from build123d import *

# Parameters (mm, degrees)
REVOLVE2_ANGLE           = 180
SKETCH5_W                = 2.54
SKETCH5_H                = 12.7
SKETCH5_W_2              = 101.6
SKETCH5_H_2              = 2.54
SKETCH5_W_3              = 12.7
BOSS_EXTRUDE1_DEPTH      = 2.54
SKETCH7_W                = 20
SKETCH7_H                = 50
CUT_EXTRUDE1_DEPTH       = 7
BOSS_EXTRUDE3_REACH      = 220.035
SKETCH8_W                = 5
SKETCH8_H                = 91.44
SKETCH9_W                = 6.129296028
SKETCH9_H                = 8.078685473
BOSS_EXTRUDE4_DEPTH      = 2
BOSS_EXTRUDE7_START      = 8
BOSS_EXTRUDE7_DEPTH      = 8
BOSS_EXTRUDE8_REACH      = 220.035
BOSS_EXTRUDE8_END_RADIUS = 40.64
SKETCH13_W               = 75.08
SKETCH13_H               = 60.08
SKETCH13_W_2             = 70
SKETCH13_H_2             = 55
SKETCH14_W               = 75.08
SKETCH14_H               = 60.08
CUT_EXTRUDE3_DEPTH       = 11
BOSS_EXTRUDE9_REACH      = 217.997
SKETCH15_W               = 70
SKETCH15_H               = 55
CUT_EXTRUDE5_DEPTH       = 15
CUT_EXTRUDE6_REACH       = 202.84
SKETCH18_W               = 12
SKETCH18_H               = 56
BOSS_EXTRUDE10_REACH     = 220.035
SKETCH23_W               = 6
SKETCH23_H               = 81.28
SKETCH26_W               = 6
SKETCH26_H               = 53.107211962
BOSS_EXTRUDE11_DEPTH     = 10


with BuildPart() as part:
    # Sketch2 → Revolve2 (revolve)
    with BuildSketch(Plane.XY):
        Polygon((0, 0), (0, 40.64), (0, 45.72), (25.4, 45.72), (195.4, 45.72), (208.1, 45.72), (208.22771659, 40.64), (195.52771659, 40.64), (25.4, 40.64), (5.08, 40.64), (5.08, 0), align=None)
    revolve(axis=Axis((0, 0, 0), (1, 0, 0)), revolution_arc=REVOLVE2_ANGLE)

    # Sketch5 → Boss-Extrude1 (add)
    with BuildSketch(Plane(origin=(0, 0, 0), x_dir=(-1, 0, 0), z_dir=(0, 0, -1))):
        with Locations((-2.54, 34.29)):
            Rectangle(SKETCH5_W, SKETCH5_H)
        with Locations((-104.113858295, -43.18)):
            Rectangle(SKETCH5_W_2, SKETCH5_H_2)
        with Locations((-11.43, 43.18)):
            Rectangle(SKETCH5_W_3, SKETCH5_H_2)
        with Locations((-104.113858295, 43.18)):
            Rectangle(SKETCH5_W_2, SKETCH5_H_2)
        with Locations((-11.43, -43.18)):
            Rectangle(SKETCH5_W_3, SKETCH5_H_2)
        with Locations((-2.54, -34.29)):
            Rectangle(SKETCH5_W, SKETCH5_H)
    extrude(amount=BOSS_EXTRUDE1_DEPTH)

    # Sketch7 → Cut-Extrude1 (cut)
    with BuildSketch(Plane.ZY):
        with Locations((10, 0)):
            Rectangle(SKETCH7_W, SKETCH7_H)
    extrude(amount=-CUT_EXTRUDE1_DEPTH, mode=Mode.SUBTRACT)

    # Sketch8 → Boss-Extrude3 (add, up to next)
    with BuildSketch(Plane(origin=(0, 0, 0), x_dir=(-1, 0, 0), z_dir=(0, 0, -1)), mode=Mode.PRIVATE) as boss_extrude3_sk1:
        with Locations((-15.58, 0)):
            Rectangle(SKETCH8_W, SKETCH8_H)
    boss_extrude3_tool1 = extrude(boss_extrude3_sk1.sketch, amount=-BOSS_EXTRUDE3_REACH, mode=Mode.PRIVATE) - part.part
    add(boss_extrude3_tool1.solids().sort_by_distance((15.58, 0, 0))[0])

    # Sketch9 → Boss-Extrude4 (add)
    with BuildSketch(Plane(origin=(5.08, 0, 0), x_dir=(0, 0, -1), z_dir=(1, 0, 0))):
        with Locations((-3.906446672, 33.952493663)):
            Rectangle(SKETCH9_W, SKETCH9_H)
    extrude(amount=BOSS_EXTRUDE4_DEPTH)

    # Sketch12 → Boss-Extrude7 (add)
    with BuildSketch(Plane.ZY.offset(-13.08).offset(BOSS_EXTRUDE7_START)):
        with BuildLine():
            Line((23.64, 33.056920607), (23.64, -33.056920607))
            ThreePointArc((23.64, -33.056920607), (40.64, 0), (23.64, 33.056920607))
        make_face()
    extrude(amount=-BOSS_EXTRUDE7_DEPTH)

    # Boss-Extrude8: up to this cylinder (the profile starts inside it)
    boss_extrude8_end = Plane(origin=(148.153858, 0, 0), z_dir=(-1, 0, 0)) * Cylinder(BOSS_EXTRUDE8_END_RADIUS, 522.35, mode=Mode.PRIVATE)
    # Sketch13 → Boss-Extrude8 (add, up to the surface)
    with BuildSketch(Plane(origin=(0, 0, 0), x_dir=(-1, 0, 0), z_dir=(0, 0, -1)), mode=Mode.PRIVATE) as boss_extrude8_sk1:
        with Locations((-148.153858295, 0)):
            Rectangle(SKETCH13_W, SKETCH13_H)
        with Locations((-148.153858295, 0)):
            Rectangle(SKETCH13_W_2, SKETCH13_H_2, mode=Mode.SUBTRACT)
    boss_extrude8_tool1 = extrude(boss_extrude8_sk1.sketch, amount=-BOSS_EXTRUDE8_REACH, mode=Mode.PRIVATE) & boss_extrude8_end
    add(boss_extrude8_tool1.solids().sort_by_distance((148.153858, 29.078407, 0))[0])

    # Sketch14 → Cut-Extrude3 (cut)
    with BuildSketch(Plane(origin=(0, 0, 0), x_dir=(-1, 0, 0), z_dir=(0, 0, -1))):
        with Locations((-148.153858295, 0)):
            Rectangle(SKETCH14_W, SKETCH14_H)
    extrude(amount=-CUT_EXTRUDE3_DEPTH, mode=Mode.SUBTRACT)

    # Sketch15 → Boss-Extrude9 (add, up to next)
    with BuildSketch(Plane(origin=(0, 0, 11), x_dir=(-1, 0, 0), z_dir=(0, 0, -1)), mode=Mode.PRIVATE) as boss_extrude9_sk1:
        with Locations((-148.153858295, 0)):
            Rectangle(SKETCH15_W, SKETCH15_H)
    boss_extrude9_tool1 = extrude(boss_extrude9_sk1.sketch, amount=-BOSS_EXTRUDE9_REACH, mode=Mode.PRIVATE) - part.part
    add(boss_extrude9_tool1.solids().sort_by_distance((148.153858, 0, 11))[0])

    # Sketch17 → Cut-Extrude5 (cut)
    with BuildSketch(Plane(origin=(0, 0, 11), x_dir=(-1, 0, 0), z_dir=(0, 0, -1))):
        Polygon((-113.153858295, 27.5), (-183.153858295, 27.5), (-183.153858295, 19.5), (-185.693858295, 19.5), (-185.693858295, 5.5), (-183.153858295, 5.5), (-183.153858295, -13.5), (-185.693858295, -13.5), (-185.693858295, -24.5), (-183.153858295, -24.5), (-183.153858295, -27.5), (-113.153858295, -27.5), align=None)
    extrude(amount=-CUT_EXTRUDE5_DEPTH, mode=Mode.SUBTRACT)

    # Sketch18 → Cut-Extrude6 (cut, up to next)
    with BuildSketch(Plane(origin=(18.08, 0, 0), x_dir=(0, 0, -1), z_dir=(1, 0, 0)), mode=Mode.PRIVATE) as cut_extrude6_sk1:
        with Locations((-6, -10.004795356)):
            Rectangle(SKETCH18_W, SKETCH18_H)
    cut_extrude6_tool1 = extrude(cut_extrude6_sk1.sketch, amount=-CUT_EXTRUDE6_REACH, mode=Mode.PRIVATE) & part.part
    add(cut_extrude6_tool1.solids().sort_by_distance((18.08, -10.004795, 6))[0], mode=Mode.SUBTRACT)

    # Sketch23 → Boss-Extrude10 (add, up to next)
    with BuildSketch(Plane(origin=(0, 0, 0), x_dir=(-1, 0, 0), z_dir=(0, 0, -1)), mode=Mode.PRIVATE) as boss_extrude10_sk1:
        with Locations((-205.22771659, 0)):
            Rectangle(SKETCH23_W, SKETCH23_H)
    boss_extrude10_tool1 = extrude(boss_extrude10_sk1.sketch, amount=-BOSS_EXTRUDE10_REACH, mode=Mode.PRIVATE) - part.part
    add(boss_extrude10_tool1.solids().sort_by_distance((205.227717, 0, 0))[0])

    # Sketch26 → Boss-Extrude11 (add)
    with BuildSketch(Plane(origin=(0, 0, 0), x_dir=(-1, 0, 0), z_dir=(0, 0, -1))):
        with Locations((-205.22771659, 39.5)):
            Rectangle(SKETCH26_W, SKETCH26_H)
    extrude(amount=BOSS_EXTRUDE11_DEPTH)


solid = part.part
Source: CAD feature listing. Evaluate the final solid. Frame: model axes, mm. A direction names the side the tool comes from. Round coordinates to 2 decimals unless told otherwise and drop trailing zeros. Loops run counter-clockwise (first coordinate to the right, second up) from the corner with the lowest first, then second, coordinate; pieces in that order, holes last.
Q1. Section A-A, the plane y = 0. Return loops of the section in (x, z), plus the area to 3 significant figures.
Q2. Mould query, pull axis Y, two halves, no side actions, for faces 4 (the face through (18.08, -1, 20)), 5 (the face through (205, 66.054, -5)), 6 (the face through (205, 12.946, -5)). Classes: pulls with the +Y half, pulls with the -Y half, needs draft (parallel to the pull), parting line crosses it, or undercut.
Q3. Ray query, line 1 (X direction, y = -9, z = 19.5); line 2 (Y direction, x = 183.5, z = 20); line 3 (X direction, y = 8, z = 21.5). Return the intervals inside material, ascending.
Q4. First-contact query: P1, Ø1.5, axis at x = 185, z = 38.5, coming from the +Y side; P2, Ø2, axis at x = 2, z = -1.5, coming from the +Y side; P3, Ø2, axis at x = 186.5, y = -27, coming from the -Z side. Flat tips, straight axial feed; report the tip coordinate or a pass-through.
Q5. Section B-B, the plane z = 17. State how many separate pieces and enclosed holes the cut face has, plus the area to 3 significant figures.
Q6. Access query for faces 1 (the face through (205, 40, -10)), 2 (the face through (112, 0, 11)), 3 (the face through (16, 17.995, 6)). Directions: +Z, -Z, +X, -X, +Y, -Y. A direction counts if a zero-diameter tool reaches every point of the face in a straight line with its end or side. Return the directions, or none.
Q7. Section C-C, the plane x = 188.5. Return loops of the section in (y, z).
Solutions:
1. outline: (0, 20) - (5.08, 20) - (5.08, 23.64) - (13.08, 23.64) - (13.08, 12) - (18.08, 12) - (18.08, 40.64) - (110.61, 40.64) - (110.61, 11) - (113.15, 11) - (113.15, 26) - (183.15, 26) - (183.15, 11) - (185.69, 11) - (185.69, 40.64) - (202.23, 40.64) - (202.23, 0) - (208.23, 0) - (208.23, 40.64) - (208.1, 45.72) - (0, 45.72) - close
1. area: 2,860 mm2
2. face 4: undercut
2. face 5: pulls with the +Y half
2. face 6: pulls with the -Y half
3. line 1: x = 13.08 to 18.08, 110.61 to 113.15, 183.15 to 185.69, 202.23 to 208.23
3. line 2: y = -41.11 to -35.38, -30.04 to -24.5, -13.5 to 5.5, 19.5 to 30.04, 35.38 to 41.11
3. line 3: x = 0 to 5.08, 13.08 to 18.08, 110.61 to 113.15, 202.23 to 208.23
4. P1: stops at y = 25.79
4. P2: stops at y = 40.64
4. P3: stops at z = 11
5. separate pieces: 3
5. enclosed holes: 1
5. area: 3,830 mm2
6. face 1: -Z, +X, -X, +Y, -Y
6. face 2: -Z
6. face 3: -Z, -X
7. outline: (-45.72, 0) - (-40.64, 0) arc R40.64 cw to (40.64, 0) - (45.72, 0) arc R45.72 ccw to start
